Geometry: see drawing. Coordinates: mm, zero at the bounding-box minimum. Coordinates: 2 decimals unless noted, no trailing zeros. Order: outer loops, then holes, each group sorted by start corner. A loop starts at its lowest first (then second) coordinate and runs counter-clockwise, first axis right, second up. Notation, with made-up numbers: M 18.25,75 L 48.25,75 A19 cw 48.25,110 Z; hole C -20.75,-12.75 d4. An arc over 180 degrees is marked long. One line per item, written item: value.
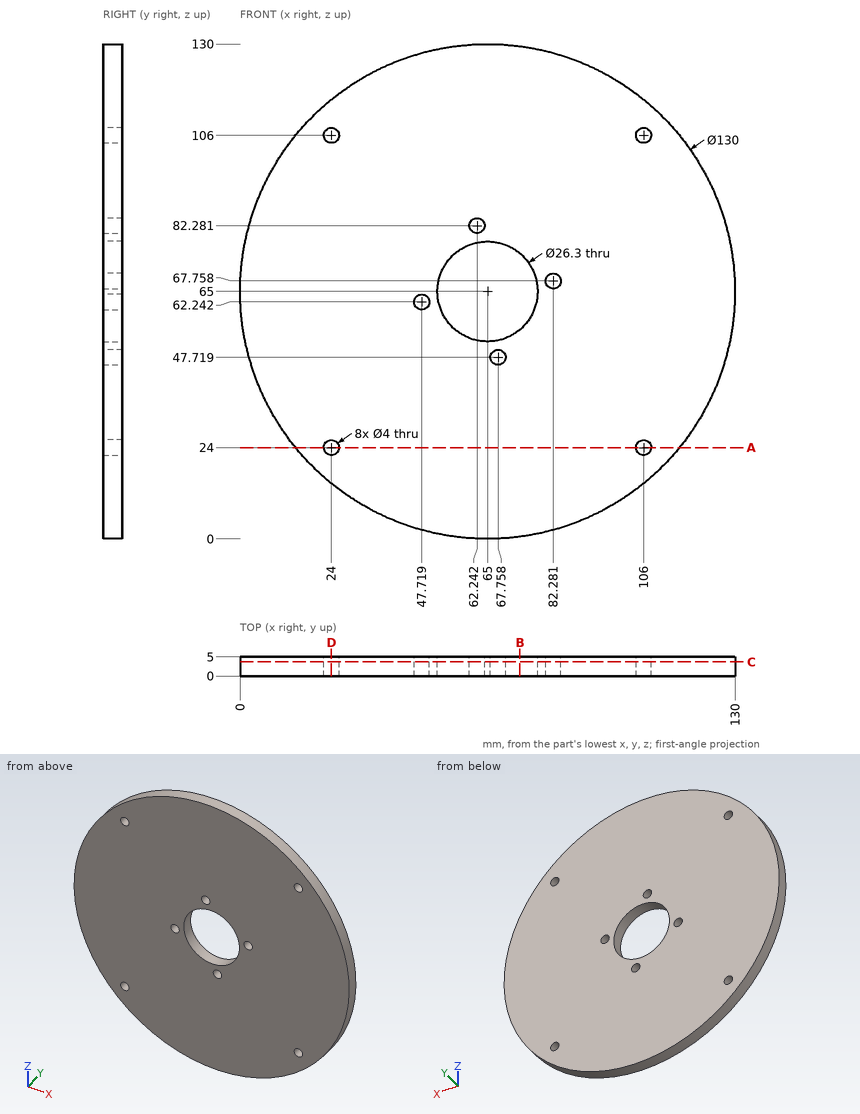
(1) Ray query, line 1 (Z direction, x = 63.5, y = 2.6) (1 decimal); line 2 (Z direction, x = 62, y = 0.5); line 3 (X direction, y = 1.3, z = 25.5). Return the intervals inside material, ascending. Write a range as from..to.
Data:
line 1: z = 0..51.9, 78.1..80.7, 83.8..130
line 2: z = 0.07..52.2, 77.8..80.3, 84.27..129.93
line 3: x = 13.38..22.68, 25.32..104.68, 107.32..116.62
(2) Cut plane C-C on y = 3.7. Give the number of separate pieces and of enclosed holes in the cut face, plus the area to 3 significant figures.
Data:
separate pieces: 1
enclosed holes: 9
area: 12,600 mm2
(3) First-contact query: pin 1 (3 mm diameter, centred on x = 52, y = 0.5, fed in from +Z) (1 decimal); pin 2 (3 mm diameter, centred on y = 2.5, z = 41.5, fed in from -X). Flat tips, straight axial feed; report the tip coordinate or a pass-through.
Data:
pin 1: stops at z = 129
pin 2: stops at x = 3.84
(4) Cut plane A-A on z = 24. Output: boundary loops of the cut face in (x, y).
Data:
outline: M 14.56,0 L 22,0 L 22,5 L 14.56,5 Z; M 26,0 L 104,0 L 104,5 L 26,5 Z; M 108,0 L 115.44,0 L 115.44,5 L 108,5 Z
(5) Cut plane D-D on x = 24. Output: boundary loops of the cut face in (y, z).
Data:
outline: M 0,14.56 L 5,14.56 L 5,22 L 0,22 Z; M 0,26 L 5,26 L 5,104 L 0,104 Z; M 0,108 L 5,108 L 5,115.44 L 0,115.44 Z
(6) Cut plane B-B on x = 73.5. Output: boundary loops of the cut face in (y, z), plus the area to 3 significant figures.
Data:
outline: M 0,0.56 L 5,0.56 L 5,54.97 L 0,54.97 Z; M 0,75.03 L 5,75.03 L 5,129.44 L 0,129.44 Z
area: 544 mm2
